Can you work these out from the drawing? Everything is in mm from the part's minimum corner. Coordinates: 2 decimals unless noted, no trailing zeros. Loops run counter-clockwise (first coordinate to the right, second up) from the corner with the lowest first, then second, coordinate; pieces in that order, holes last.
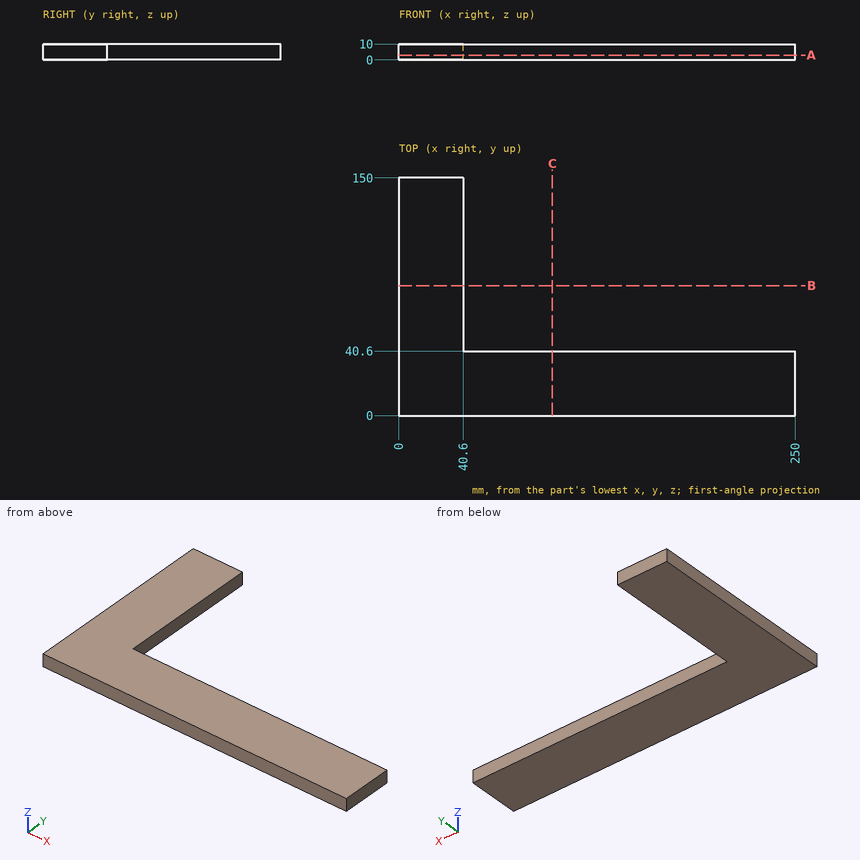
1. I want a section at A-A (z = 3). Please give me the cut outline in (x, y).
2. I need wall thicknesses on line 1 along Y through (x, z) = (143.5, 2.5). Which ranges of the line are inside material? Lowest first, please.
3. For pin 1 (4 mm diameter, centred on x = 102.5, z = 4.5, fed in from +Y); pin 2 (5 mm diameter, centred on y = 114, z = 7, fed in from +X), each with a flat end and sliding along its axis, tell me the tip position at first contact or that it passes through.
4. I want a section at B-B (y = 82). Please give me the cut outline in (x, z).
Response values:
1. outline: (0, 0) - (250, 0) - (250, 40.6) - (40.6, 40.6) - (40.6, 150) - (0, 150) - close
2. line 1: y = 0 to 40.6
3. pin 1: stops at y = 40.6
3. pin 2: stops at x = 40.6
4. outline: (0, 0) - (40.6, 0) - (40.6, 10) - (0, 10) - close
